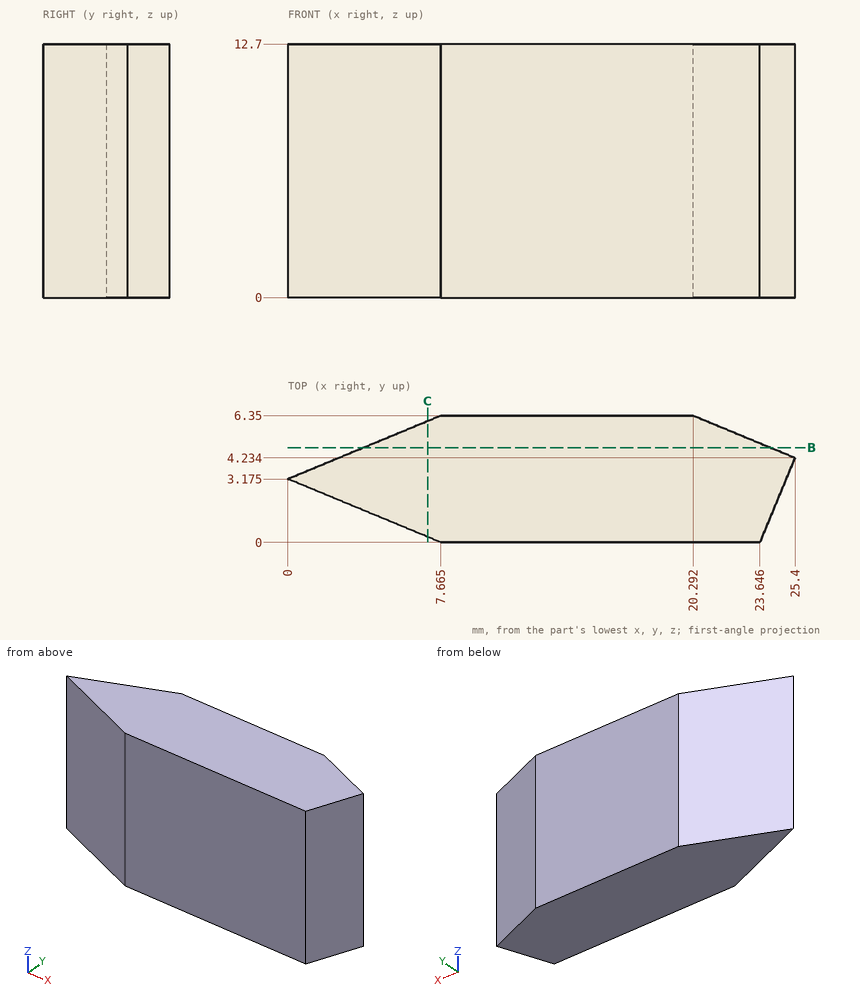
Job drawing, mm, ordinate dimensions from the low corner. One solid piece. Coordinates: 2 decimals unless noted, no trailing zeros. Order: outer loops, then holes, each group sorted by start corner. A loop starts at its lowest first (then second) coordinate and runs counter-clockwise, first axis right, second up. Notation, with made-up numbers: M 37,82 L 41,82 A19 cw 41,106 Z; hole C 63,40 d1. An arc over 180 degrees is marked long. Answer as CSV lines item,"result".
(1) Wall check: line 1 along X through (y, z) = (2, 9.25) (1 decimal); line 2 along Y through (x, z) = (2, 7.25); line 3 along X through (y, z) = (2.25, 7) (1 decimal). Give the ranges that are in metal, low to high.
Geometry says:
line 1,"x = 2.8 to 24.5"
line 2,"y = 2.35 to 4"
line 3,"x = 2.2 to 24.6"
(2) Band-saw the part on B-B, the plane y = 4.75. List the corners of the cut face in (x, z) (1 decimal).
Geometry says:
outline,"M 3.8,0 L 24.2,0 L 24.2,12.7 L 3.8,12.7 Z"
(3) Band-saw the part on C-C, the plane x = 7. List the corners of the cut face in (y, z).
Geometry says:
outline,"M 0.28,0 L 6.07,0 L 6.07,12.7 L 0.28,12.7 Z"
(4) Flat gauge pins, fed straight in: pin 1 (3 mm diameter, centred on y = 5.5, z = 10, fed in from +X); pin 2 (1 mm diameter, centred on y = 5.5, z = 5.5, fed in from -X) (1 decimal). Where does each tip first touch, or does it go through?
Geometry says:
pin 1,"stops at x = 25.4"
pin 2,"stops at x = 4.4"
